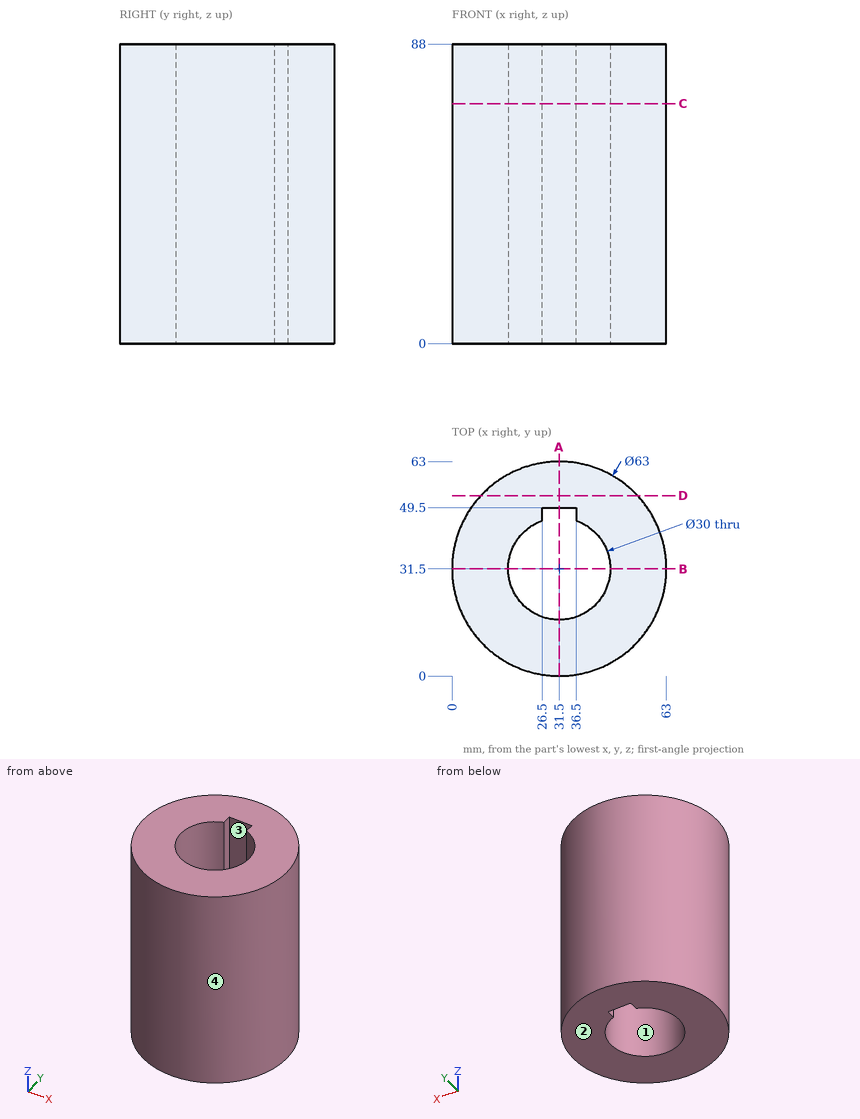
Study the drawing (mm; zero at the part's minimum x, y, z) and answer. Round coordinates to 2 decimals unless told otherwise and drop trailing zeros. Order: outer loops, then holes, each group sorted by start corner. A loop starts at its lowest first (then second) coordinate and runs counter-clockwise, first axis right, second up. Notation, with made-up numbers: (-32.75, 88) -> (-24.75, 88) arc R11 ccw to (-24.75, 106) -> close; hole circle Ø9 at (-34.75, 29.25). An arc over 180 degrees is marked (long way). Answer as CSV lines item,"result". Start each with the question number.
(1) The part is cut by section B-B (y = 31.5). Determine the outline of the cut face in (x, z), then the cut area to 3 significant figures.
(2) The part is cut by section C-C (z = 70.5). Determine the outline of the cut face in (x, y).
(3) Flat-ended cylindrical pins translate along their axes: pin 1 Ø5 at (x, z) = (30.5, 37.5) entering from -Y; pin 2 Ø10 at (x, z) = (53, 52.5) entering from -Y; pin 3 Ø1 at (y, z) = (16, 64) entering from -X. Find the tip coordinate at first contact, or state that the pin passes through.
(4) For a pull along Y with two mould halves and no side action, classify the marked faces 1, 2, 3 and 4 as +Y half, -Y half, draft (parallel to the pull), parting line (faces both ways), or undercut.
(5) Find the intervals of material crossed by probe 1 along X at (y, z) = (31, 46); probe 2 along Y at (x, z) = (32, 38); probe 3 along X at (y, z) = (37, 53.5), in increasing order. Write a range as from..to.
(6) The part is cut by section D-D (y = 53). Determine the outline of the cut face in (x, z).
(7) The part is cut by section A-A (x = 31.5). Determine the outline of the cut face in (y, z), then the cut area to 3 significant figures.
Evaluation:
1,outline,"(0, 0) -> (16.5, 0) -> (16.5, 88) -> (0, 88) -> close; (46.5, 0) -> (63, 0) -> (63, 88) -> (46.5, 88) -> close"
1,area,"2,900 mm²"
2,outline,"circle Ø63 at (31.5, 31.5); hole (26.5, 45.64) arc R15 ccw (long way) to (36.5, 45.64) -> (36.5, 49.5) -> (26.5, 49.5) -> close"
3,pin 1,"y = 0"
3,pin 2,"y = 4.67"
3,pin 3,"x = 3.8"
4,face 1,"undercut"
4,face 2,"draft"
4,face 3,"undercut"
4,face 4,"parting line"
5,probe 1,"0..16.51, 46.49..63"
5,probe 2,"0..16.51, 49.5..63"
5,probe 3,"0.48..17.54, 45.46..62.52"
6,outline,"(8.48, 0) -> (54.52, 0) -> (54.52, 88) -> (8.48, 88) -> close"
7,outline,"(0, 0) -> (16.5, 0) -> (16.5, 88) -> (0, 88) -> close; (49.5, 0) -> (63, 0) -> (63, 88) -> (49.5, 88) -> close"
7,area,"2,640 mm²"
